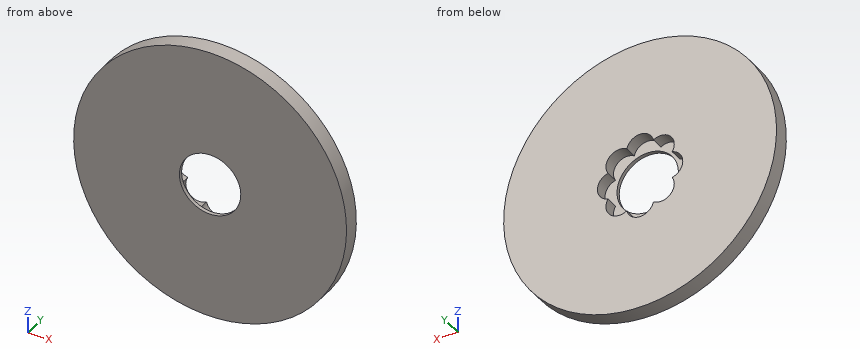
```python
from build123d import *

# Parameters (mm, degrees)
SKETCH1_R           = 100
BOSS_EXTRUDE1_DEPTH = 12
SKETCH2_R           = 22.5
CUT_EXTRUDE1_DEPTH  = 142.929559994
SKETCH3_R           = 10
CUT_EXTRUDE2_DEPTH  = 9.274253
CIRPATTERN1_START   = 2.725746995
CIRPATTERN1_DEPTH   = 9.274253005


# Read off the part's stored shape, not the designer's step: CirPattern1
with BuildPart() as part:
    # Sketch1 → Boss-Extrude1 (new body)
    with BuildSketch(Plane(origin=(0, 0, 0), x_dir=(1, 0, 0), z_dir=(0, 1, 0))):
        with Locations(Location((0, 0, 0), (0, 0, 270))):
            Circle(SKETCH1_R)
    extrude(amount=BOSS_EXTRUDE1_DEPTH)

    # Sketch2 → Cut-Extrude1 (cut, through all)
    with BuildSketch(Plane(origin=(0, 0, 0), x_dir=(1, 0, 0), z_dir=(0, 1, 0))):
        with Locations(Location((0, 0, 0), (0, 0, 270))):
            Circle(SKETCH2_R)
    extrude(amount=CUT_EXTRUDE1_DEPTH, mode=Mode.SUBTRACT)

    # Sketch3 → Cut-Extrude2 (cut)
    with BuildSketch(Plane(origin=(0, 12, 0), x_dir=(1, 0, 0), z_dir=(0, 1, 0))):
        with Locations((-21.277260677, 0)):
            Circle(SKETCH3_R)
    extrude(amount=-CUT_EXTRUDE2_DEPTH, mode=Mode.SUBTRACT)

    # CirPattern1 outline → CirPattern1 (cut)
    with BuildSketch(Plane(origin=(0, 0, 0), x_dir=(1, 0, 0), z_dir=(0, 1, 0)).offset(CIRPATTERN1_START)):
        with BuildLine():
            ThreePointArc((-20.185206991, -9.940192088), (-21.863151487, -9.982821843), (-23.524589593, -9.744204059))
            ThreePointArc((-23.524589593, -9.744204059), (-22.116363122, -22.116363122), (-9.744204059, -23.524589593))
            ThreePointArc((-9.744204059, -23.524589593), (0, -31.277260677), (9.744204059, -23.524589593))
            ThreePointArc((9.744204059, -23.524589593), (22.116363122, -22.116363122), (23.524589593, -9.744204059))
            ThreePointArc((23.524589593, -9.744204059), (31.277260677, 0), (23.524589593, 9.744204059))
            ThreePointArc((23.524589593, 9.744204059), (22.116363122, 22.116363122), (9.744204059, 23.524589593))
            ThreePointArc((9.744204059, 23.524589593), (0, 31.277260677), (-9.744204059, 23.524589593))
            ThreePointArc((-9.744204059, 23.524589593), (-22.116363122, 22.116363122), (-23.524589593, 9.744204059))
            ThreePointArc((-23.524589593, 9.744204059), (-21.863151487, 9.982821843), (-20.185206991, 9.940192088))
            ThreePointArc((-20.185206991, 9.940192088), (22.5, 0), (-20.185206991, -9.940192088))
        make_face()
    extrude(amount=CIRPATTERN1_DEPTH, mode=Mode.SUBTRACT)


solid = part.part
```
The model under review builds one solid part; all positions refer to its coordinate system, in mm. Round coordinates to 2 decimals unless told otherwise and drop trailing zeros. Write each loop counter-clockwise with the first axis right and the second up, starting at its lowest first coordinate (ties: lowest second). Pieces come first, ordered by that corner, then holes.
(1) We need section A-A on z = 0. Give the boundary of the cut face in (x, y), and give its area (3 significant figures).
(2) We need section D-D on z = -28.5. Give the boundary of the cut face in (x, y).
(3) Insertion check: pin 1 (1.5 mm diameter, centred on x = -4.5, y = 10, fed in from -Z); pin 2 (5 mm diameter, centred on y = 8.5, z = -64.5, fed in from +X); pin 3 (4 mm diameter, centred on x = -54.5, y = 2.5, fed in from +Z). Each pin has a flat end and moves straight along its axis. Give the tip position at first contact, or say it passes through.
(4) We need section C-C on y = 6. Give the boundary of the cut face in (x, z), and give its area (3 significant figures).
(5) We need section B-B on x = 0. Give the boundary of the cut face in (y, z).
(6) Wall thickness on L1, parallel to X at y = 2.1, z = 0; L2, parallel to X at y = 2, z = 20.5; L3, parallel to Z at x = -27.5, y = 9: over which ranges is each line inside the solid? List them lowest first.
Findings below:
1. outline: (-100, 0) - (-22.5, 0) - (-22.5, 2.73) - (-31.28, 2.73) - (-31.28, 12) - (-100, 12) - close; (22.5, 0) - (100, 0) - (100, 12) - (31.28, 12) - (31.28, 2.73) - (22.5, 2.73) - close
1. area: 1,700 mm2
2. outline: (-95.85, 0) - (95.85, 0) - (95.85, 12) - (6.92, 12) - (6.92, 2.73) - (-6.92, 2.73) - (-6.92, 12) - (-95.85, 12) - close
3. pin 1: stops at z = -99.93
3. pin 2: stops at x = 78.46
3. pin 3: stops at z = 85.11
4. outline: circle Ø200 at (0, 0); hole (-23.52, -9.74) arc R10 ccw to (-9.74, -23.52) arc R10 ccw to (9.74, -23.52) arc R10 ccw to (23.52, -9.74) arc R10 ccw to (23.52, 9.74) arc R10 ccw to (9.74, 23.52) arc R10 ccw to (-9.74, 23.52) arc R10 ccw to (-23.52, 9.74) arc R10 ccw to start
4. area: 28,700 mm2
5. outline: (0, -100) - (12, -100) - (12, -31.28) - (2.73, -31.28) - (2.73, -22.5) - (0, -22.5) - close; (0, 22.5) - (2.73, 22.5) - (2.73, 31.28) - (12, 31.28) - (12, 100) - (0, 100) - close
6. L1: x = -100 to -22.5, 22.5 to 100
6. L2: x = -97.88 to -9.27, 9.27 to 97.88
6. L3: z = -96.14 to -7.83, 7.83 to 96.14
